Part model, mm, in its own coordinate system. Face numbers are marked on the shaded views. A direction names the side the tool comes from. Coordinates: 2 decimals unless noted, no trailing zeros. Loops run counter-clockwise (first coordinate to the right, second up) from the corner with the lowest first, then second, coordinate; pieces in that order, holes last. Notation, with made-up numbers: M 24,80 L 33,80 A19 cw 33,106 Z; hole C -35.5,56 d4. An arc over 180 degrees is marked long. Use CSV: the item, a comma, the result in double quotes. Start each with the question number.
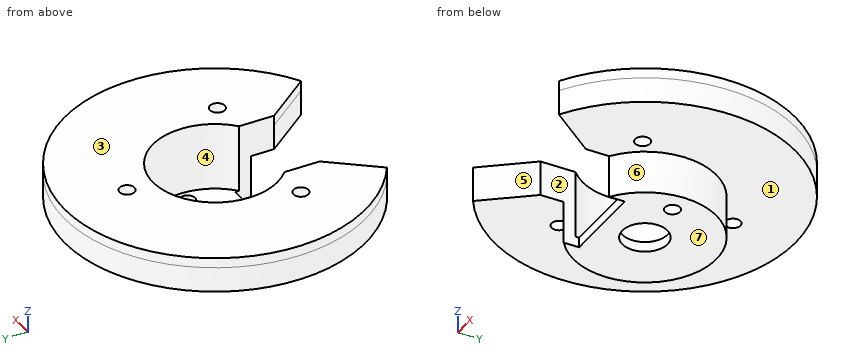
from build123d import *

# Parameters (mm, degrees)
SKETCH_1_R               = 14.25
SKETCH_1_R_2             = 12.4
EXTRUDE_1_DEPTH          = 13.5
EXTRUDE_START            = 2
SKETCH_2_R               = 14.25
SKETCH_2_R_2             = 4.5
SKETCH_2_R_3             = 1.5
EXTRUDE_2_DEPTH          = 2
EXTRUDE_START_2          = -2
SKETCH_5_R               = 30
SKETCH_5_R_2             = 12.4
EXTRUDE_3_DEPTH          = 2
CUT_EXTRUDE_2_DEPTH      = 2
CUT_EXTRUDE_2_DEPTH_BACK = 19
SKETCH_6_R               = 1.5
CUT_EXTRUDE_3_DEPTH      = 2
SKETCH_8_R               = 1.5
EXTRUDE_4_DEPTH          = 5


with BuildPart() as part:
    # 草图1 → 凸台-拉伸1 (new body)
    with BuildSketch(Plane.XY):
        Circle(SKETCH_1_R)
        Circle(SKETCH_1_R_2, mode=Mode.SUBTRACT)
    extrude(amount=EXTRUDE_1_DEPTH)

    # 草图2 → 凸台-拉伸2 (add)
    with BuildSketch(Plane(origin=(0, 0, 0), x_dir=(-1, 0, 0), z_dir=(0, 0, -1)).offset(EXTRUDE_START)):
        Circle(SKETCH_2_R)
        Circle(SKETCH_2_R_2, mode=Mode.SUBTRACT)
        with Locations((-10, 0)):
            Circle(SKETCH_2_R_3, mode=Mode.SUBTRACT)
    extrude(amount=-EXTRUDE_2_DEPTH)

    # 草图5 → 凸台-拉伸3 (add)
    with BuildSketch(Plane.XY.offset(13.5).offset(EXTRUDE_START_2)):
        Circle(SKETCH_5_R)
        Circle(SKETCH_5_R_2, mode=Mode.SUBTRACT)
    extrude(amount=EXTRUDE_3_DEPTH)

    # 草图4 → 切除-拉伸2 (cut, two sides: drawn at the far end of the back side and taken through both)
    with BuildSketch(Plane.XY.offset(13.5).offset(-CUT_EXTRUDE_2_DEPTH_BACK)):
        Polygon((-8.25, -16.255900921), (-15.579618383, -25.637384637), (-4.242821572, -33.778563125), (18.383281344, -29.225909584), (8.25, -16.255900921), (8.25, -8.544099079), (-8.25, -8.544099079), align=None)
    extrude(amount=CUT_EXTRUDE_2_DEPTH + CUT_EXTRUDE_2_DEPTH_BACK, mode=Mode.SUBTRACT)

    # 草图6 → 切除-拉伸3 (cut)
    with BuildSketch(Plane.XY.offset(13.5)):
        with Locations((0, 17.5)):
            Circle(SKETCH_6_R)
        with Locations((15.155444566, -8.75)):
            Circle(SKETCH_6_R)
        with Locations((-15.155444566, -8.75)):
            Circle(SKETCH_6_R)
    extrude(amount=-CUT_EXTRUDE_3_DEPTH, mode=Mode.SUBTRACT)

    # 草图8 → 凸台-拉伸4 (add)
    with BuildSketch(Plane(origin=(0, 0, 11.5), x_dir=(-1, 0, 0), z_dir=(0, 0, -1))):
        with BuildLine():
            Line((8.25, -11.618950039), (8.25, -16.255900921))
            Line((8.25, -16.255900921), (15.579618383, -25.637384637))
            ThreePointArc((15.579618383, -25.637384637), (0, 30), (-15.579618383, -25.637384637))
            Line((-15.579618383, -25.637384637), (-8.25, -16.255900921))
            Line((-8.25, -16.255900921), (-8.25, -11.618950039))
            ThreePointArc((-8.25, -11.618950039), (0, 14.25), (8.25, -11.618950039))
        make_face()
        with Locations(Location((0, 17.5, 0), (0, 0, 180))):
            Circle(SKETCH_8_R, mode=Mode.SUBTRACT)
        with Locations(Location((-15.155444566, -8.75, 0), (0, 0, 180))):
            Circle(SKETCH_8_R, mode=Mode.SUBTRACT)
        with Locations(Location((15.155444566, -8.75, 0), (0, 0, 180))):
            Circle(SKETCH_8_R, mode=Mode.SUBTRACT)
    extrude(amount=EXTRUDE_4_DEPTH)


solid = part.part
1. Pin check, flat tips, straight feed: pin 1 (2 mm diameter, centred on y = 10.5, z = 11, fed in from +X); pin 2 (1 mm diameter, centred on x = 4, z = -1, fed in from -Y); pin 3 (5 mm diameter, centred on x = 15.16, y = -8.75, fed in from -Z); pin 4 (20 mm diameter, centred on x = 0, y = 0, fed in from -Z). Stop position of each tip, or through.
2. Wall check: probe 1 along X at (y, z) = (-8.75, 9.1); probe 2 along Z at (x, y) = (20.5, -18); probe 3 along X at (y, z) = (-13.5, 7.5). Give the ranges that are in metal, low to high.
3. Slice it at A-A, the plane x = 0. List the corners of the cut face in (y, z).
4. Slice it at D-D, the plane y = 17.5. List the corners of the cut face in (x, z).
5. Tool access for the marked faces 1, 2 and 3: list every direction of +Z, -Z, +X, -X, +Y, -Y with a clear straight run to the whole face (end or side of a thin tool).
6. Slice it at C-C, the plane z = 7.5. List the corners of the cut face in (x, y), and give its area (3 significant figures).
7. Two-plate mould, pull along Y, no slides. Class the marked faces 4, 5, 6 and 7: pulls with the +Y half, pulls with the -Y half, needs draft (parallel to the pull), parting line crosses it, or undercut.
8. Slice it at B-B, the plane y = 0. List the corners of the cut face in (x, z), and give its area (3 significant figures).
Found:
1,pin 1,"x = 28.46"
1,pin 2,"y = -8.54"
1,pin 3,"z = 6.5"
1,pin 4,"z = -2"
2,probe 1,"-28.7 to -16.66, -13.66 to -8.79, 8.79 to 13.66, 16.66 to 28.7"
2,probe 2,"6.5 to 13.5"
2,probe 3,"-26.79 to -8.25, 8.25 to 26.79"
3,outline,"M -8.54,-2 L -4.5,-2 L -4.5,0 L -8.54,0 Z; M 4.5,-2 L 14.25,-2 L 14.25,6.5 L 16,6.5 L 16,13.5 L 12.4,13.5 L 12.4,0 L 4.5,0 Z; M 19,6.5 L 30,6.5 L 30,13.5 L 19,13.5 Z"
4,outline,"M -24.37,6.5 L -1.5,6.5 L -1.5,13.5 L -24.37,13.5 Z; M 1.5,6.5 L 24.37,6.5 L 24.37,13.5 L 1.5,13.5 Z"
5,face 1,"-Z"
5,face 2,"+Z, -Z, -Y"
5,face 3,"+Z, +X, -X, +Y, -Y"
6,outline,"M -15.58,-25.64 L -8.25,-16.26 L -8.25,-9.26 A12.4 cw long 8.25,-9.26 L 8.25,-16.26 L 15.58,-25.64 A30 ccw long Z; hole C -15.16,-8.75 d3; hole C 0,17.5 d3; hole C 15.16,-8.75 d3"
6,area,"1,930 mm^2"
7,face 4,"undercut"
7,face 5,"pulls with the -Y half"
7,face 6,"parting line crosses it"
7,face 7,"needs draft"
8,outline,"M -30,6.5 L -14.25,6.5 L -14.25,-2 L -4.5,-2 L -4.5,0 L -12.4,0 L -12.4,13.5 L -30,13.5 Z; M 4.5,-2 L 8.5,-2 L 8.5,0 L 4.5,0 Z; M 11.5,-2 L 14.25,-2 L 14.25,6.5 L 30,6.5 L 30,13.5 L 12.4,13.5 L 12.4,0 L 11.5,0 Z"
8,area,"303 mm^2"
